Verification items for the finished model (mm, model axes). Give positions to 0.01 mm unless a question says otherwise; leave off trailing zeros. Write each loop counter-clockwise with the first axis right and the second up, starting at its lowest first coordinate (ties: lowest second). Pieces come first, ordered by that corner, then holes. Notation, with made-up numbers: (34.5, -34.75) - (59.5, -34.75) arc R12 ccw to (59.5, -23.75) - close; hole circle Ø3 at (62.25, 7). An arc over 180 degrees is marked (long way). Put each result on its own line as item: value.
from build123d import *

# Parameters (mm, degrees)
SKETCH1_W           = 50
SKETCH1_H           = 100
BOSS_EXTRUDE1_DEPTH = 2262.74
SKETCH2_W           = 50
SKETCH2_H           = 70.027066898
BOSS_EXTRUDE2_DEPTH = 1
SKETCH3_W           = 50
SKETCH3_H           = 42.703513447
BOSS_EXTRUDE3_DEPTH = 1
SKETCH4_R           = 5
CUT_EXTRUDE1_DEPTH  = 309
SKETCH7_R           = 12.5
CUT_EXTRUDE2_DEPTH  = 100
BOSS_EXTRUDE5_DEPTH = 50


with BuildPart() as part:
    # Sketch1 → Boss-Extrude1 (new body)
    with BuildSketch(Plane.XY):
        with Locations((25, 50)):
            Rectangle(SKETCH1_W, SKETCH1_H)
    extrude(amount=BOSS_EXTRUDE1_DEPTH)

    # Sketch2 → Boss-Extrude2 (add)
    with BuildSketch(Plane(origin=(0, 100, 0), x_dir=(1, 0, 0), z_dir=(0, 1, 0))):
        with Locations((25, -35.013533449)):
            Rectangle(SKETCH2_W, SKETCH2_H)
    extrude(amount=BOSS_EXTRUDE2_DEPTH)

    # Sketch3 → Boss-Extrude3 (add)
    with BuildSketch(Plane.XZ):
        with Locations((25, 732.888243277)):
            Rectangle(SKETCH3_W, SKETCH3_H)
    extrude(amount=BOSS_EXTRUDE3_DEPTH)

    # Sketch4 → Cut-Extrude1 (cut)
    with BuildSketch(Plane(origin=(50, 0, 0), x_dir=(0, 0, -1), z_dir=(1, 0, 0))):
        with Locations((-732.888243277, 51.05890277)):
            Circle(SKETCH4_R)
    extrude(amount=-CUT_EXTRUDE1_DEPTH, mode=Mode.SUBTRACT)

    # Sketch7 → Cut-Extrude2 (cut)
    with BuildSketch(Plane.ZY):
        with Locations((62.269457415, 50.5)):
            Circle(SKETCH7_R)
    extrude(amount=-CUT_EXTRUDE2_DEPTH, mode=Mode.SUBTRACT)

    # Sketch8 → Boss-Extrude5 (add)
    with BuildSketch(Plane(origin=(50, 0, 0), x_dir=(0, 0, -1), z_dir=(1, 0, 0))):
        Polygon((-2262.74, 0), (-2351.764948591, 0), (-2262.74, 100), align=None)
    extrude(amount=-BOSS_EXTRUDE5_DEPTH)


solid = part.part
Q1. Section check B-B, the plane z = 1483. Record the cut outline in (x, y), plus the area to 3 significant figures.
Answers follow:
outline: (0, 0) - (50, 0) - (50, 100) - (0, 100) - close
area: 5,000 mm2
Q2. Go/stop test with flat-tipped pins: pin 1 Ø6 at (x, y) = (34.5, 43) entering from -Z; pin 2 Ø0.5 at (x, y) = (29, -0.5) entering from +Z; pin 3 Ø3 at (x, z) = (33, 655.5) entering from -Y; pin 4 Ø12 at (x, z) = (37.5, 1306.5) entering from +Y. Record where each tip stops, or that it passes through.
Answers follow:
pin 1: stops at z = 0
pin 2: stops at z = 754.24
pin 3: stops at y = 0
pin 4: stops at y = 100
Q3. Section check A-A, the plane x = 31. Record the cut outline in (y, z).
Answers follow:
outline: (-1, 711.54) - (0, 711.54) - (0, 0) - (101, 0) - (101, 70.03) - (100, 70.03) - (100, 2262.74) - (0, 2351.76) - (0, 754.24) - (-1, 754.24) - close; hole circle Ø25 at (50.5, 62.27); hole circle Ø10 at (51.06, 732.89)
Q4. Scan lines: line 1 along Z through (x, y) = (15, 50); line 2 along Z through (x, y) = (15.5, 53.5); line 3 along Y through (x, z) = (23.5, 1200). Record each from-to range of solid material in increasing order.
Answers follow:
line 1: z = 0 to 49.78, 74.76 to 728, 737.77 to 2307.25
line 2: z = 0 to 50.13, 74.4 to 728.52, 737.25 to 2304.14
line 3: y = 0 to 100
